For this review, use the dimensioned drawing (mm, ordinates from the lowest corner) and the shaded views. Coordinates: 2 decimals unless noted, no trailing zeros. Loops run counter-clockwise (first coordinate to the right, second up) from the corner with the lowest first, then second, coordinate; pieces in that order, holes last. Notation, with made-up numbers: (35.5, -2) -> (91.5, -2) arc R22 ccw to (91.5, 16) -> close; hole circle Ø4 at (-5.5, 4). An arc over 180 degrees is marked (long way). Answer as a JSON object with one key per item and string values.
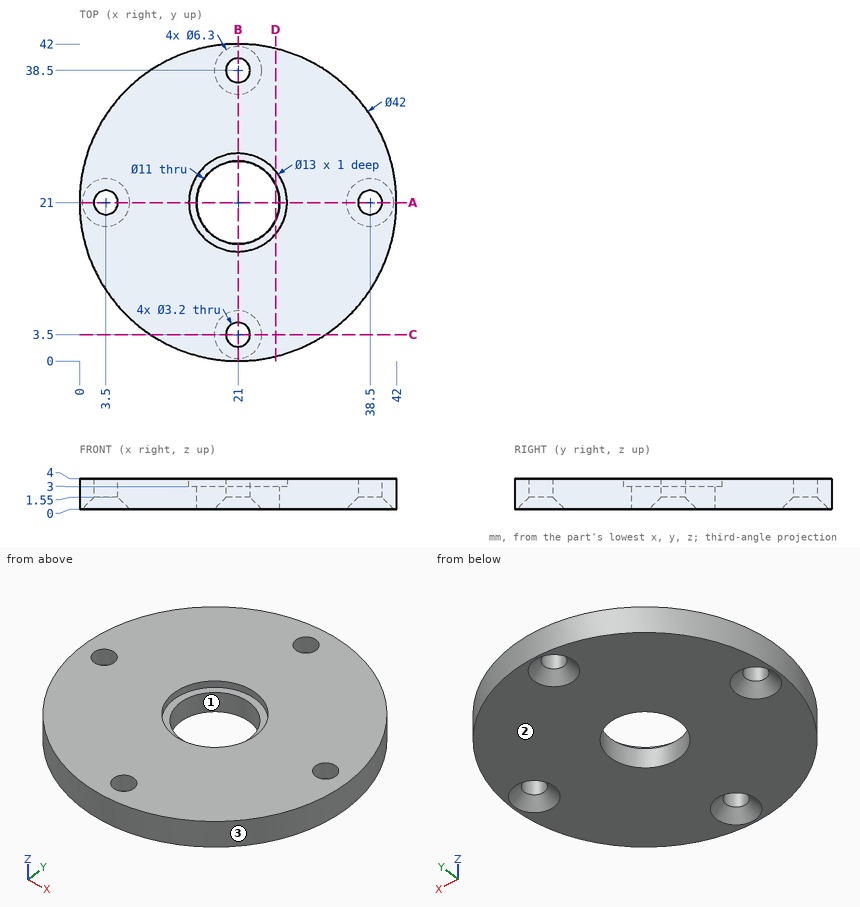
1) Clearance check with flat-ended pins moving along their axes: pin 1 Ø6.5 at (x, y) = (19.5, 18.5) entering from +Z; pin 2 Ø1.5 at (y, z) = (30.5, 0.5) entering from +X. State where each tip first meets the part, or that it passes through.
Completed:
{"pin 1": "z = 3", "pin 2": "x = 40.09"}
2) The part is to be moulded in two halves that separate along X. For the marked faces 1, 2 and 3, say which applies: pulls with the +X half, pulls with the -X half, needs draft (parallel to the pull), parting line crosses it, or undercut.
Completed:
{"face 1": "undercut", "face 2": "needs draft", "face 3": "parting line crosses it"}
3) Add section C-C, the plane y = 3.5. Give the boundary of the cut face in (x, z), and give its area (3 significant figures).
Completed:
{"outline": "(9.39, 0) -> (17.85, 0) -> (19.4, 1.55) -> (19.4, 4) -> (9.39, 4) -> close; (22.6, 1.55) -> (24.15, 0) -> (32.61, 0) -> (32.61, 4) -> (22.6, 4) -> close", "area": "77.7 mm²"}
4) Add section A-A, the plane y = 21. Give the boundary of the cut face in (x, z).
Completed:
{"outline": "(0, 0) -> (0.35, 0) -> (1.9, 1.55) -> (1.9, 4) -> (0, 4) -> close; (5.1, 1.55) -> (6.65, 0) -> (15.5, 0) -> (15.5, 3) -> (14.5, 3) -> (14.5, 4) -> (5.1, 4) -> close; (26.5, 0) -> (35.35, 0) -> (36.9, 1.55) -> (36.9, 4) -> (27.5, 4) -> (27.5, 3) -> (26.5, 3) -> close; (40.1, 1.55) -> (41.65, 0) -> (42, 0) -> (42, 4) -> (40.1, 4) -> close"}
5) Wall thickness on probe 1 along Y at (x, z) = (21, 1.6); probe 2 along Y at (x, z) = (22.5, 0.7); probe 3 along Z at (x, y) = (16, 25): over which ranges is each line inside the solid? List them lowest first.
Completed:
{"probe 1": "0 to 1.9, 5.1 to 15.5, 26.5 to 36.9, 40.1 to 42", "probe 2": "0.05 to 1.56, 5.44 to 15.71, 26.29 to 36.56, 40.44 to 41.95", "probe 3": "0 to 3"}
6) Add section D-D, the plane x = 26. Give the boundary of the cut face in (y, z).
Completed:
{"outline": "(0.6, 0) -> (18.71, 0) -> (18.71, 3) -> (16.85, 3) -> (16.85, 4) -> (0.6, 4) -> close; (23.29, 0) -> (41.4, 0) -> (41.4, 4) -> (25.15, 4) -> (25.15, 3) -> (23.29, 3) -> close"}
